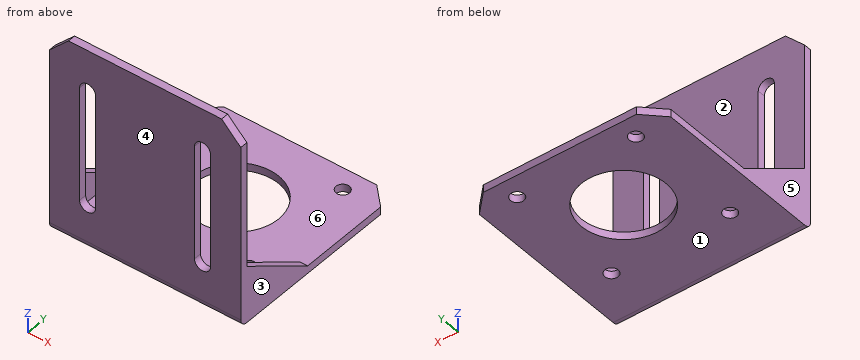
Autodesk Inventor part; units mm, degrees
ref_plane "YZ Plane" through (0, 0, 0) normal (1, 0, 0) x (0, 1, 0)
ref_plane "XZ Plane" through (0, 0, 0) normal (0, 1, 0) x (-1, 0, 0)
ref_plane "XY Plane" through (0, 0, 0) normal (0, 0, 1) x (1, 0, 0)
sketch "Boceto1" plane through (0, 0, 0) normal (0, 0, 1) x (1, 0, 0)
  line L0 (0, 0) -> (50, 0)
  line L1 (50, 0) -> (50, 46)
  line L2 (45, 51) -> (5, 51)
  line L3 (0, 46) -> (0, 0)
  circle A0 centre (25, 30) radius 11.05
  line L4 (5, 51) -> (0, 46)
  line L5 (50, 46) -> (45, 51)
  point P0 (50, 51)
  point P1 (0, 51)
  point P2 (25, 0)
  point P3 (9.5, 45.5)
  point P4 (40.5, 45.5)
  point P5 (9.5, 14.5)
  point P6 (40.5, 14.5)
  dimension "d0" = 50
  dimension "d1" = 51
  dimension "d2" = 21
  dimension "d3" = 22.1
  dimension "d15" = 5
  dimension "d16" = 5
  dimension "d17" = 5
  dimension "d18" = 5
  dimension "d50" = 15.5
  dimension "d51" = 15.5
  dimension "d54" = 31
  dimension "d57" = 31
extrude "Extrusión1" add sketch "Boceto1" along normal blind 2
sketch "Boceto2" plane through (0, 0, 0) normal (0, -1, 0) x (1, 0, 0)
  line L0 (50, 2) -> (0, 2)
  line L1 (0, 0) -> (0, 2)
  line L2 (0, 0) -> (50, 0)
  line L3 (50, 0) -> (50, 2)
  line L4 (0, 0) -> (0, 48)
  line L5 (5, 53) -> (45, 53)
  line L6 (50, 48) -> (50, 0)
  line L7 (10, 44.1) -> (10, 44.1)
  line L8 (12.1, 42) -> (12.1, 12)
  line L9 (10, 9.9) -> (10, 9.9)
  line L10 (7.9, 12) -> (7.9, 42)
  arc A0 (10, 44.1) -> (7.9, 42) centre (10, 42) ccw
  arc A1 (12.1, 42) -> (10, 44.1) centre (10, 42) ccw
  arc A2 (7.9, 12) -> (10, 9.9) centre (10, 12) ccw
  arc A3 (10, 9.9) -> (12.1, 12) centre (10, 12) ccw
  line L11 (40, 44.1) -> (40, 44.1)
  line L12 (42.1, 42) -> (42.1, 12)
  line L13 (40, 9.9) -> (40, 9.9)
  line L14 (37.9, 12) -> (37.9, 42)
  arc A4 (40, 44.1) -> (37.9, 42) centre (40, 42) ccw
  arc A5 (42.1, 42) -> (40, 44.1) centre (40, 42) ccw
  arc A6 (37.9, 12) -> (40, 9.9) centre (40, 12) ccw
  arc A7 (40, 9.9) -> (42.1, 12) centre (40, 12) ccw
  line L15 (0, 48) -> (5, 53)
  line L16 (45, 53) -> (50, 48)
  point P0 (0, 53)
  point P1 (50, 53)
  point P2 (7.9, 44.1)
  point P3 (12.1, 44.1)
  point P4 (7.9, 9.9)
  point P5 (37.9, 44.1)
  point P6 (42.1, 44.1)
  point P7 (37.9, 9.9)
  dimension "d21" = 53
  dimension "d24" = 4.2
  dimension "d25" = 7.9
  dimension "d26" = 2.1
  dimension "d27" = 2.1
  dimension "d30" = 30
  dimension "d37" = 5
  dimension "d38" = 5
  dimension "d39" = 5
  dimension "d40" = 5
  dimension "d67" = 30
  dimension "d68" = 11
extrude "Extrusión2" add sketch "Boceto2" against normal blind 2 contours L0 L4 L15 L5 L16 L6
sketch "Boceto3" plane through (50, 0, 0) normal (1, 0, 0) x (0, 0, -1)
  line L0 (-2, 46) -> (-2, 2)
  line L1 (-2, 2) -> (-48, 2)
  line L2 (-2, 2) -> (-2, 22)
  line L3 (-2, 22) -> (-15, 2)
  line L4 (-15, 2) -> (-2, 2)
  dimension "d41" = 20
  dimension "d42" = 13
extrude "Extrusión3" add sketch "Boceto3" against normal blind 2
pattern_linear "Patrón rectangular1" count 2 spacing 48 along (-1, 0, 0) of "Extrusión3"
fillet "Empalme1" radius 2 1 edges at (25, 2, 2)
fillet "Empalme2" radius 2 1 edges at (25, 0, 0)
hole "Hole1" at (9.5, 45.5, 0) at (40.5, 45.5, 0) at (9.5, 14.5, 0) at (40.5, 14.5, 0) direction (0, 0, 1) diameter 3.5 end through all
properties part number "NEMA17Support"
Source: CAD feature listing. Evaluate the final solid. Frame: model axes, mm. Face numbers are marked on the shaded views. A direction names the side the tool comes from. Round coordinates to 2 decimals unless told otherwise and drop trailing zeros. Write each loop counter-clockwise with the first axis right and the second up, starting at its lowest first coordinate (ties: lowest second). Pieces come first, ordered by that corner, then holes. Notation, with made-up numbers: M -7.5,75 L 22.5,75 A19 ccw 22.5,89 Z; hole C -36,-29 d3. An arc over 180 degrees is marked long. One line per item, written item: value. Start each with the question number.
Item 1: Set-up query: the marked faces 1 and 2. Return all of +Z, -Z, +X, -X, +Y, -Y with unobstructed straight access to the full face (end or side cutting, diameter ignored); none if empty.
Item 2: Pin query (flat end, axial travel): pin 1 (14.5 mm diameter, centred on x = 19.5, z = 37.5, fed in from +Y); pin 2 (14 mm diameter, centred on x = 19.5, y = 18, fed in from +Z). Return the tip coordinate at first contact, or that it passes through.
Item 3: Mould query, pull axis X, two halves, no side actions, for the marked faces 3, 4, 5 and 6. Classes: pulls with the +X half, pulls with the -X half, needs draft (parallel to the pull), parting line crosses it, or undercut.
Item 4: Section query B-B (y = 24). Return the cut outline in (x, z), plus the area to 3 significant figures.
Item 5: Ray query, L1, parallel to X at y = 14.5, z = 1.05; L2, parallel to Y at x = 9.5, z = 1.05; L3, parallel to X at y = 9, z = 3. Return the intervals inside material, ascending. Write a range as from..to.
Item 6: Section query A-A (x = 18.5). Return the cut outline in (y, z), plus the area to 3 significant figures.
Item 7: Section query C-C (x = 9.5). Return the cut outline in (y, z).
Item 8: Section query D-D (z = 11). Return the cut outline in (x, y).
Result set:
1. face 1: -Z, +X, -X, +Y, -Y
1. face 2: +Z, +Y
2. pin 1: stops at y = 2
2. pin 2: stops at z = 2
3. face 3: pulls with the +X half
3. face 4: needs draft
3. face 5: pulls with the -X half
3. face 6: undercut
4. outline: M 0,0 L 15.72,0 L 15.72,2 L 0,2 Z; M 34.28,0 L 50,0 L 50,2 L 34.28,2 Z
4. area: 62.9 mm²
5. L1: x = 0..7.75, 11.25..38.75, 42.25..50
5. L2: y = 0.24..12.75, 16.25..43.75, 47.25..51
5. L3: x = 0..2, 48..50
6. outline: M 0,2 A2 ccw 2,0 L 21.06,0 L 21.06,2 L 4,2 A2 cw 2,4 L 2,53 L 0,53 Z; M 38.94,0 L 51,0 L 51,2 L 38.94,2 Z
6. area: 168 mm²
7. outline: M 0,2 A2 ccw 2,0 L 12.75,0 L 12.75,2 L 4,2 A2 cw 2,4 L 2,9.96 L 0,9.96 Z; M 0,44.04 L 2,44.04 L 2,53 L 0,53 Z; M 16.25,0 L 43.75,0 L 43.75,2 L 16.25,2 Z; M 47.25,0 L 51,0 L 51,2 L 47.25,2 Z
8. outline: M 0,0 L 8.15,0 L 8.15,2 L 2,2 L 2,8.15 L 0,8.15 Z; M 11.85,0 L 38.15,0 L 38.15,2 L 11.85,2 Z; M 41.85,0 L 50,0 L 50,8.15 L 48,8.15 L 48,2 L 41.85,2 Z
